Build history of the part. All positions in model axes, mm. Face numbers are marked on the shaded views. Round coordinates to 2 decimals unless told otherwise and drop trailing zeros. Loops run counter-clockwise (first coordinate to the right, second up) from the corner with the lowest first, then second, coordinate; pieces in that order, holes last.
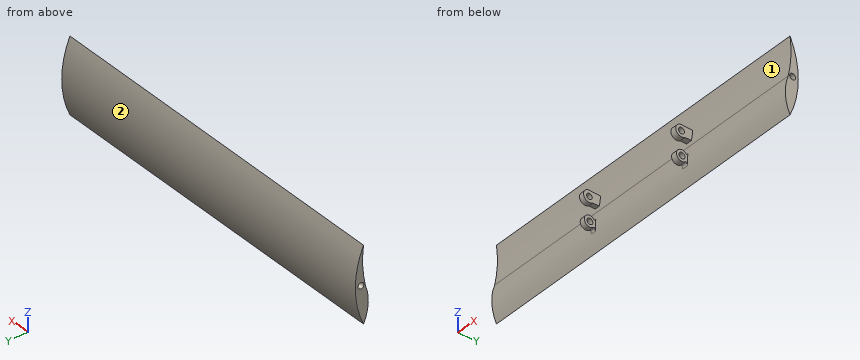
from build123d import *

# Parameters (mm, degrees)
BOSS_EXTRUDE2_DEPTH = 1200
SKETCH4_R           = 10
CUT_EXTRUDE2_DEPTH  = 30
SKETCH5_R           = 10
BOSS_EXTRUDE3_DEPTH = 20
SCALE1_SCALE        = 0.15
SKETCH8_R           = 1.423275346
SKETCH8_R_2         = 1.5
BOSS_EXTRUDE4_DEPTH = 2.5


with BuildPart() as part:
    # Sketch2 → Boss-Extrude2 (new body)
    with BuildSketch(Plane(origin=(0, 0, 0), x_dir=(0, 0, -1), z_dir=(1, 0, 0))):
        with BuildLine():
            ThreePointArc((-77.006621836, 0), (47.993378164, 27.282197134), (172.993378164, 0))
            ThreePointArc((172.993378164, 0), (113.40797201, -15.816647718), (52.515991285, -6.18577782))
            ThreePointArc((52.515991285, -6.18577782), (-11.973891604, 2.590390407), (-77.006621836, 0))
        make_face()
    extrude(amount=BOSS_EXTRUDE2_DEPTH)

    # Sketch4 → Cut-Extrude2 (cut)
    with BuildSketch(Plane.ZY):
        with Locations((-47.993378164, 8.438388981)):
            Circle(SKETCH4_R)
    cut_extrude2 = extrude(amount=-CUT_EXTRUDE2_DEPTH, mode=Mode.SUBTRACT)

    # Mirror1: Cut-Extrude2 across plane
    add(cut_extrude2.mirror(Plane(origin=(600, 0, 0), x_dir=(0, 0, 1), z_dir=(1, 0, 0))), mode=Mode.SUBTRACT)

    # Sketch5 → Boss-Extrude3 (add)
    with BuildSketch(Plane(origin=(800, 0, 0), x_dir=(0, 0, -1), z_dir=(1, 0, 0))):
        with BuildLine():
            Line((81.410704846, -14.011940423), (85.13998826, -17.780929187))
            ThreePointArc((85.13998826, -17.780929187), (85.592469343, -18.332508198), (85.935038434, -18.958307649))
            ThreePointArc((85.935038434, -18.958307649), (94.512681221, -52.437390339), (110.389076807, -21.739426291))
            ThreePointArc((110.389076807, -21.739426291), (109.883111494, -19.399677201), (111.633319944, -17.766521641))
            Line((111.633319944, -17.766521641), (119.894685982, -15.3415971))
            Line((119.894685982, -15.3415971), (121.619163907, -14.881341581))
            ThreePointArc((121.619163907, -14.881341581), (101.241742119, -14.900548765), (80.905670019, -13.602912771))
            Line((80.905670019, -13.602912771), (81.410704846, -14.011940423))
        make_face()
        with Locations((96.602298961, -34.063635389)):
            Circle(SKETCH5_R, mode=Mode.SUBTRACT)
        with BuildLine():
            Line((0, 1.824950196), (0, -28.482665363))
            ThreePointArc((0, -28.482665363), (20.687062812, -54.790757496), (34.369104077, -24.247803704))
            Line((34.369104077, -24.247803704), (34.369104077, -2.546400914))
            ThreePointArc((34.369104077, -2.546400914), (17.235436494, 0.039346175), (0, 1.824950196))
        make_face()
        with Locations((18.091069948, -35.85231876)):
            Circle(SKETCH5_R, mode=Mode.SUBTRACT)
    extrude(amount=-BOSS_EXTRUDE3_DEPTH)


with BuildPart() as part_1:
    # Scale1: scaled about (601.252748222, 6.649777436, -64.506234279)
    add(part.part.scale(SCALE1_SCALE).moved(Location((511.064835989, 5.652310821, -54.830299137))))

    # Sketch8 → Boss-Extrude4 (add)
    with BuildSketch(Plane(origin=(572.064835989, 0, 0), x_dir=(0, 0, -1), z_dir=(1, 0, 0))):
        with BuildLine():
            Line((54.830299137, 5.92605335), (54.830299137, 1.379911016))
            ThreePointArc((54.830299137, 1.379911016), (57.933358559, -2.566302804), (59.985664749, 2.015140265))
            Line((59.985664749, 2.015140265), (59.985664749, 5.270350684))
            Line((59.985664749, 5.270350684), (56.48845574, 5.92605335))
            Line((56.48845574, 5.92605335), (54.830299137, 5.92605335))
        make_face()
        with Locations((57.574663837, 0.344776051)):
            Circle(SKETCH8_R, mode=Mode.SUBTRACT)
        with BuildLine():
            Line((67.041904864, 3.550519757), (67.669169538, 2.902434591))
            Line((67.669169538, 2.902434591), (67.720554902, 2.808564673))
            ThreePointArc((67.720554902, 2.808564673), (69.00720132, -2.21329773), (71.388660658, 2.391396877))
            ThreePointArc((71.388660658, 2.391396877), (71.312765861, 2.742359241), (71.575297129, 2.987332575))
            Line((71.575297129, 2.987332575), (72.814502034, 3.351071256))
            ThreePointArc((72.814502034, 3.351071256), (69.921739963, 3.263724136), (67.041904864, 3.550519757))
        make_face()
        with Locations((69.320643981, 0.542765513)):
            Circle(SKETCH8_R_2, mode=Mode.SUBTRACT)
    extrude(amount=BOSS_EXTRUDE4_DEPTH)


solid = part_1.part
(1) Probe line 1 (X direction, y = 2.5, z = -58.5); line 2 (Y direction, x = 520.5, z = -53.5); line 3 (Y direction, x = 663, z = -71). List the from-to ranges inside material, lowest first.
Responses:
line 1: x = 572.06 to 574.56, 628.06 to 631.06
line 2: y = 6.02 to 8.93
line 3: y = 3.25 to 8.84
(2) Slice it at A-A on x = 646. List the corners of the cut face in (y, z).
Responses:
outline: (4.72, -62.71) arc R22.37 ccw to (5.65, -80.78) arc R45 ccw to (5.65, -43.28) arc R55.84 cw to start
(3) Slice it at C-C on z = -50. List the corners of the cut face in (x, y), plus the area to 3 significant figures.
Responses:
outline: (511.06, 6.1) - (691.06, 6.1) - (691.06, 8.11) - (511.06, 8.11) - close
area: 361 mm2
(4) Pin check, flat tips, straight feed: P1, Ø6.5, axis at y = 0, z = -59, coming from the -X side; P2, Ø3.5, axis at y = 0.54, z = -69.32, coming from the +X side; P3, Ø5, axis at x = 663.5, z = -67, coming from the -Y side; P4, Ø2.5, axis at y = 0.27, z = -57.54, coming from the -X side. Stop position of each tip, or through.
Responses:
P1: stops at x = 572.06
P2: stops at x = 631.06
P3: stops at y = 3.28
P4: passes through
(5) Slice it at B-B on z = -78. List the corners of the cut face in (x, y), plus the area to 3 significant figures.
Responses:
outline: (511.06, 4.48) - (691.06, 4.48) - (691.06, 6.82) - (511.06, 6.82) - close
area: 421 mm2
(6) Pull direction Z, two halves, no side cores. Call the marked faces 1 and 2: +Z half, -Z half, draft (parallel to the pull), parting line (faces both ways), or undercut.
Responses:
face 1: undercut
face 2: parting line
